The model under review builds one solid part; all positions refer to its coordinate system, in mm. Coordinates: 2 decimals unless noted, no trailing zeros. Write each loop counter-clockwise with the first axis right and the second up, starting at its lowest first coordinate (ties: lowest second). Pieces come first, ordered by that corner, then holes. Notation, with made-up numbers: M 28,-23 L 33,-23 A17 cw 33,-10 Z; hole C -3,-21.75 d2. An arc over 180 degrees is marked long. Answer as a JSON object with one key per item and string values.
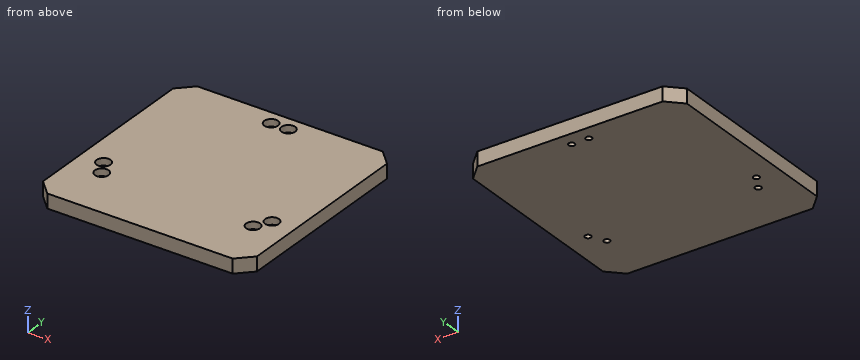
```python
from build123d import *

# Parameters (mm, degrees)
F0_W           = 150
F0_H           = 150
F1_DEPTH       = 10
F3_D           = 4.2
F3_DEPTH       = 15.8
F3_CBORE_D     = 9.75
F3_CBORE_DEPTH = 5
F3_TIP         = 1.2618073
F4_SIZE        = 10


with BuildPart() as f1:
    # F0 (on Top) → F1 (new body)
    with BuildSketch(Plane.XY):
        Rectangle(F0_W, F0_H)
    extrude(amount=F1_DEPTH)

    # F3
    with Locations(Plane.XY.offset(10)):
        with Locations((-6, 64.7224845011), (6, 64.7224845011), (-59.051315774, -27.1650898279), (-53.051315774, -37.5573946733), (53.051315774, -37.5573946733), (59.051315774, -27.1650898279)):
            CounterBoreHole(F3_D / 2, F3_CBORE_D / 2, F3_CBORE_DEPTH, depth=F3_DEPTH)
            with Locations((0, 0, -(F3_DEPTH + F3_TIP / 2))):  # 118° drill point
                Cone(0, F3_D / 2, F3_TIP, mode=Mode.SUBTRACT)

    # F4
    f4_edges = [f1.edges().sort_by_distance(p)[0] for p in [
        (-75, 75, 5),
        (75, 75, 5),
        (75, -75, 5),
        (-75, -75, 5),
    ]]
    chamfer(f4_edges, length=F4_SIZE)


solid = f1.part
```
(1) Add section A-A on x = 6. Give the boundary of the cut face in (y, z).
Results list:
{"outline": "M -75,0 L 62.62,0 L 62.62,5 L 59.85,5 L 59.85,10 L -75,10 Z; M 66.82,0 L 75,0 L 75,10 L 69.6,10 L 69.6,5 L 66.82,5 Z"}
(2) Wall thickness on line 1 along Y through (x, z) = (6, 8.55); line 2 along Y through (x, z) = (6, 2.6); line 3 along X through (y, z) = (64, 9.75): over which ranges is each line inside the solid? List them lowest first. Write a range as from..to.
Results list:
{"line 1": "-75..59.85, 69.6..75", "line 2": "-75..62.62, 66.82..75", "line 3": "-75..-10.82, -1.18..1.18, 10.82..75"}
(3) Add section B-B on z = 6.75. Give the boundary of the cut face in (x, y) (3 decimals), and give its area (3 significant figures).
Results list:
{"outline": "M -75,-65 L -65,-75 L 65,-75 L 75,-65 L 75,65 L 65,75 L -65,75 L -75,65 Z; hole C -59.051,-27.165 d9.75; hole C -53.051,-37.557 d9.75; hole C -6,64.722 d9.75; hole C 6,64.722 d9.75; hole C 53.051,-37.557 d9.75; hole C 59.051,-27.165 d9.75", "area": "21,900 mm²"}
(4) For pin 1 Ø3 at (x, y) = (51, -38.5) entering from +Z, flat-tipped, find the tip position at first contact; note if it passes through.
Results list:
{"pin 1": "z = 5"}
